Read the model definition and answer for the solid it produces. Units are mm, in the model's axes. A direction names the side the tool comes from. Coordinates: 2 decimals unless noted, no trailing zeros. Order: outer loops, then holes, each group sorted by start corner. A loop starts at its lowest first (then second) coordinate and runs counter-clockwise, first axis right, second up. Notation, with made-up numbers: M -27.5,21.5 L -4.5,21.5 A9 ccw -4.5,27.5 Z; hole C 75,10.25 d10. An arc over 180 degrees is marked long. Use a Markdown table: item, result. Add a question column.
1) The mould has two halves that part along X. Classify faces 3 (the face through (-50.48, 46.61, -21.04)), 4 (the face through (-26.15, 87.218, -26.038)), 5 (the face through (-9.352, 54.274, -25.475)): released by +X, released by -X, zero draft, split by the parting line, or undercut.
2) Find the intervals of material crossed by probe 1 along X at (y, z) = (87.5, -24.5); probe 2 along Y at (x, z) = (-34.5, -22.75); probe 3 along Z at (x, y) = (-10, 94), in increasing order. Write a range as [from, to].
3) Find section B-B on z = -21.5. Write down the section's boundary in (x, y), plus the area to 3 significant figures.
4) Each of these flat-tipped pins is pushed along its axis until it touches: pin 1 Ø5 at (x, y) = (-19, 80.5) entering from -Z; pin 2 Ø5 at (x, y) = (-16.08, 55.44) entering from -Z; pin 3 Ø3 at (x, z) = (-44, -26.5) entering from -Y. Where does it stop, or does it pass through?
5) Find section A-A on z = -27. Write down the section's boundary in (x, y).
6) For faces 1 (the face through (-14.835, 58.443, -23.065)), 2 (the face through (-9.314, 87.768, -25.475)), determine the directions among +Z, -Z, +X, -X, +Y, -Y from which every point of the face is accessible in a straight line to the end or side of a thin tool.
Autodesk Inventor part; units mm, degrees
ref_plane "YZ Plane" through (0, 0, 0) normal (1, 0, 0) x (0, 1, 0)
ref_plane "XZ Plane" through (0, 0, 0) normal (0, 1, 0) x (-1, 0, 0)
ref_plane "XY Plane" through (0, 0, 0) normal (0, 0, 1) x (1, 0, 0)
ref_plane "Arbeitsebene15" through (-38.58009, 58.540516, -23.010083) normal (0, 0, 1) x (1, 0, 0)
sketch "Skizze38" plane through (-38.58009, 58.540516, -23.010083) normal (0, 0, 1) x (1, 0, 0)
  circle A0 centre (27, 33.3) radius 3
  circle A1 centre (-8.3, 27) radius 3
  circle A2 centre (-2, -8.3) radius 3
  circle A3 centre (33.3, -2) radius 3
  circle A4 centre (27, -8.3) radius 3
  circle A5 centre (-8.3, -2) radius 3
  circle A6 centre (-2, 33.3) radius 3
  circle A7 centre (33.3, 27) radius 3
  line L0 (27.5, 29.5) -> (-2.5, 29.5)
  arc A8 (29.5, 27.5) -> (27.5, 29.5) centre (27.5, 27.5) ccw
  line L1 (29.5, 27.5) -> (29.5, -2.5)
  arc A9 (27.5, -4.5) -> (29.5, -2.5) centre (27.5, -2.5) ccw
  line L2 (-2.5, -4.5) -> (27.5, -4.5)
  arc A10 (-4.5, -2.5) -> (-2.5, -4.5) centre (-2.5, -2.5) ccw
  line L3 (-4.5, -2.5) -> (-4.5, 27.5)
  arc A11 (-2.5, 29.5) -> (-4.5, 27.5) centre (-2.5, 27.5) ccw
  circle A12 centre (33.5, 33.5) radius 2.5
  circle A13 centre (-8.5, -8.5) radius 2.5
  circle A14 centre (33.5, -8.5) radius 2.5
  circle A15 centre (-8.5, 33.5) radius 2.5
  line L4 (-11.75, -10.5) -> (-11.75, 8.25)
  arc A16 (-11.75, -10.5) -> (-10.5, -11.75) centre (-10.5, -10.5) ccw
  line L5 (8.25, -11.75) -> (-10.5, -11.75)
  line L6 (8.25, -13.877389) -> (8.25, -11.75)
  arc A17 (7.405556, -14.865216) -> (8.25, -13.877389) centre (7.25, -13.877389) ccw
  arc A18 (7.405556, -14.865216) -> (7.6, -17.35) centre (7.6, -16.1) ccw
  line L7 (17.4, -17.35) -> (7.6, -17.35)
  arc A19 (17.4, -17.35) -> (17.594444, -14.865216) centre (17.4, -16.1) ccw
  arc A20 (16.75, -13.877389) -> (17.594444, -14.865216) centre (17.75, -13.877389) ccw
  line L8 (16.75, -11.75) -> (16.75, -13.877389)
  line L9 (35.5, -11.75) -> (16.75, -11.75)
  arc A21 (35.5, -11.75) -> (36.75, -10.5) centre (35.5, -10.5) ccw
  line L10 (36.75, 6.487451) -> (36.75, -10.5)
  arc A22 (36.75, 6.487451) -> (36.55605, 6.521706) centre (36.65, 6.487451) ccw
  arc A23 (31.3, 7.45) -> (36.55605, 6.521706) centre (34.01, 7.45) ccw
  line L11 (31.3, 17.55) -> (31.3, 7.45)
  arc A24 (36.55605, 18.478294) -> (31.3, 17.55) centre (34.01, 17.55) ccw
  arc A25 (36.55605, 18.478294) -> (36.75, 18.512549) centre (36.65, 18.512549) ccw
  line L12 (36.75, 35.5) -> (36.75, 18.512549)
  arc A26 (36.75, 35.5) -> (35.5, 36.75) centre (35.5, 35.5) ccw
  line L13 (18.512549, 36.75) -> (35.5, 36.75)
  arc A27 (18.512549, 36.75) -> (18.478294, 36.55605) centre (18.512549, 36.65) ccw
  arc A28 (17.55, 31.3) -> (18.478294, 36.55605) centre (17.55, 34.01) ccw
  line L14 (7.45, 31.3) -> (17.55, 31.3)
  arc A29 (6.521706, 36.55605) -> (7.45, 31.3) centre (7.45, 34.01) ccw
  arc A30 (6.521706, 36.55605) -> (6.487451, 36.75) centre (6.487451, 36.65) ccw
  line L15 (-10.5, 36.75) -> (6.487451, 36.75)
  arc A31 (-10.5, 36.75) -> (-11.75, 35.5) centre (-10.5, 35.5) ccw
  line L16 (-11.75, 16.75) -> (-11.75, 35.5)
  line L17 (-13.877389, 16.75) -> (-11.75, 16.75)
  arc A32 (-14.865216, 17.594444) -> (-13.877389, 16.75) centre (-13.877389, 17.75) ccw
  arc A33 (-14.865216, 17.594444) -> (-17.35, 17.4) centre (-16.1, 17.4) ccw
  line L18 (-17.35, 7.6) -> (-17.35, 17.4)
  arc A34 (-17.35, 7.6) -> (-14.865216, 7.405556) centre (-16.1, 7.6) ccw
  arc A35 (-13.877389, 8.25) -> (-14.865216, 7.405556) centre (-13.877389, 7.25) ccw
  line L19 (-11.75, 8.25) -> (-13.877389, 8.25)
  line L20 (-2.5, 30.1) -> (27.5, 30.1)
  arc A36 (30.1, 27.5) -> (27.5, 30.1) centre (27.5, 27.5) ccw
  line L21 (30.1, 27.5) -> (30.1, -2.5)
  arc A37 (27.5, -5.1) -> (30.1, -2.5) centre (27.5, -2.5) ccw
  line L22 (27.5, -5.1) -> (-2.5, -5.1)
  arc A38 (-5.1, -2.5) -> (-2.5, -5.1) centre (-2.5, -2.5) ccw
  line L23 (-5.1, -2.5) -> (-5.1, 27.5)
  arc A39 (-2.5, 30.1) -> (-5.1, 27.5) centre (-2.5, 27.5) ccw
  point P0 (38.58009, -58.540516)
  dimension "d425" = 0.6
sketch "Skizze38 outline for Extrusion20" plane through (-38.58009, 58.540516, -23.010083) normal (0, 0, 1) x (1, 0, 0)
  arc A0 (-5.1, -2.5) -> (-2.5, -5.1) centre (-2.5, -2.5) ccw
  line L0 (-5.1, 27.5) -> (-5.1, -2.5)
  arc A1 (-2.5, 30.1) -> (-5.1, 27.5) centre (-2.5, 27.5) ccw
  line L1 (27.5, 30.1) -> (-2.5, 30.1)
  arc A2 (30.1, 27.5) -> (27.5, 30.1) centre (27.5, 27.5) ccw
  line L2 (30.1, -2.5) -> (30.1, 27.5)
  arc A3 (27.5, -5.1) -> (30.1, -2.5) centre (27.5, -2.5) ccw
  line L3 (-2.5, -5.1) -> (27.5, -5.1)
extrude "Extrusion20" add sketch "Skizze38 outline for Extrusion20" against normal blind 5 draft -3
sketch "Skizze39" plane through (-38.58009, 58.540516, -23.010083) normal (0, 0, 1) x (1, 0, 0)
  line L0 (-2.5, -5.1) -> (27.5, -5.1)
  arc A0 (27.5, -5.1) -> (30.1, -2.5) centre (27.5, -2.5) ccw
  line L1 (30.1, -2.5) -> (30.1, 27.5)
  arc A1 (30.1, 27.5) -> (27.5, 30.1) centre (27.5, 27.5) ccw
  line L2 (27.5, 30.1) -> (-2.5, 30.1)
  arc A2 (-2.5, 30.1) -> (-5.1, 27.5) centre (-2.5, 27.5) ccw
  line L3 (-5.1, 27.5) -> (-5.1, -2.5)
  arc A3 (-5.1, -2.5) -> (-2.5, -5.1) centre (-2.5, -2.5) ccw
  line L4 (17.5, -12.5) -> (35.5, -12.5)
  line L5 (-10.5, 37.5) -> (35.5, 37.5)
  line L6 (37.5, 35.5) -> (37.5, -10.5)
  line L7 (35.5, -12.5) -> (-10.5, -12.5)
  line L8 (-12.5, -10.5) -> (-12.5, 35.5)
  line L9 (-12.5, 37.5) -> (37.5, -12.5) construction
  line L10 (37.5, 37.5) -> (-12.5, -12.5) construction
  arc A4 (37.5, 35.5) -> (35.5, 37.5) centre (35.5, 35.5) ccw
  arc A5 (37.5, 35.5) -> (35.5, 37.5) centre (35.5, 35.5) ccw
  arc A6 (-10.5, 37.5) -> (-12.5, 35.5) centre (-10.5, 35.5) ccw
  arc A7 (-12.5, -10.5) -> (-10.5, -12.5) centre (-10.5, -10.5) ccw
  arc A8 (35.5, -12.5) -> (37.5, -10.5) centre (35.5, -10.5) ccw
  point P0 (38.58009, -58.540516)
  point P1 (12.5, 12.5)
  point P2 (35.5, -12.5)
  dimension "d428" = 50
  dimension "d429" = 50
  dimension "d430" = 2
extrude "Extrusion21" add sketch "Skizze39" along normal blind 4 contours A3 L3 A2 L2 A1 L1 A0 L0 | L7 A7 L8 A6 L5 A4 L6 A8 L4
sketch "Skizze40" plane through (-38.58009, 58.540516, -19.010083) normal (0, 0, 1) x (1, 0, 0)
  arc A0 (-10.5, 37.5) -> (-12.5, 35.5) centre (-10.5, 35.5) ccw
  line L0 (-12.5, 35.5) -> (-12.5, -10.5)
  arc A1 (-12.5, -10.5) -> (-10.5, -12.5) centre (-10.5, -10.5) ccw
  line L1 (-10.5, -12.5) -> (35.5, -12.5)
  arc A2 (35.5, -12.5) -> (37.5, -10.5) centre (35.5, -10.5) ccw
  line L2 (37.5, -10.5) -> (37.5, 35.5)
  arc A3 (37.5, 35.5) -> (35.5, 37.5) centre (35.5, 35.5) ccw
  line L3 (35.5, 37.5) -> (-10.5, 37.5)
  circle A4 centre (12.5, 12.5) radius 5
  line L4 (-2.5, 20) -> (27.5, 20) construction
  line L5 (27.5, 20) -> (27.5, -8) construction
  line L6 (27.5, -8) -> (-2.5, -8) construction
  line L7 (-2.5, -8) -> (-2.5, 20) construction
  circle A5 centre (2.5, -3.1) radius 1.5
  circle A6 centre (22.5, -3.1) radius 1.5
  point P0 (38.58009, -58.540516)
  dimension "d433" = 10
  dimension "d434" = 30
  dimension "d435" = 28
  dimension "d436" = 15
  dimension "d437" = 25
  dimension "d438" = 25
  dimension "d439" = 7.5
  dimension "d440" = 3
  dimension "d441" = 3
  dimension "d442" = 5
  dimension "d443" = 5
  dimension "d466" = 15.6
  dimension "d467" = 15.6
extrude "Extrusion22" cut sketch "Skizze40" against normal through all contours A4 | A5 | A6
sketch "Skizze41" plane through (-38.58009, 58.540516, -28.010083) normal (0, 0, -1) x (-1, 0, 0)
  circle A0 centre (-12.5, 12.5) radius 5
  circle A1 centre (-4.5, 28.5) radius 1.4
  circle A2 centre (-20.5, 28.5) radius 1.4
  circle A3 centre (-2.5, -3.1) radius 1.5
  circle A4 centre (-22.5, -3.1) radius 1.5
  point P0 (-38.58009, -58.540516)
  point P1 (-3.17813, -4.837961)
  point P2 (-1.82187, -4.837961)
  point P3 (-23.17813, -4.837961)
  point P4 (-21.82187, -4.837961)
  dimension "d456" = 2.8
  dimension "d457" = 2.8
  dimension "d458" = 16
  dimension "d459" = 16
  dimension "d460" = 8
  dimension "d461" = 8
hole "Bohrung10" at (-34.08009, 87.040516, -28.010083) at (-18.08009, 87.040516, -28.010083) at (-36.08009, 55.440516, -28.010083) at (-16.08009, 55.440516, -28.010083) direction (0, 0, 1) diameter 2.8 end through all counterbore diameter 6.5 counterbore depth 8
ref_plane "Arbeitsebene16" through (-38.58009, 58.540516, -24.010083) normal (0, 0, -1) x (-1, 0, 0)
sketch "Skizze44" plane through (-38.58009, 58.540516, -24.010083) normal (0, 0, -1) x (-1, 0, 0)
  circle A0 centre (-12.5, 12.5) radius 5
  circle A1 centre (-12.5, 12.5) radius 16
  point P0 (-38.58009, -58.540516)
  dimension "d472" = 32
extrude "Extrusion25" cut sketch "Skizze44" along normal through all draft 5 contours A0 | A1
equation "\"d_i\" = 40"
equation "\"d_o\" = 40"
equation "\"d_part\" = 50"
equation "\"d6\" = 0"
equation "\"d7\" = 0"
equation "\"d8\" = 0"
equation "\"d9\" = 0"
equation "\"d13\" = 0"
equation "\"d14\" = 0"
equation "\"d20\" = 0"
equation "\"d21\" = 0"
equation "\"d22\" = 0"
equation "\"d23\" = 0"
equation "\"d24\" = 0"
equation "\"d25\" = 3"
equation "\"d26\" = 0"
equation "\"d27\" = 0"
equation "\"d28\" = 0"
equation "\"d29\" = 0"
equation "\"d30\" = 0"
equation "\"d31\" = 0"
equation "\"d32\" = 0"
equation "\"d33\" = 0"
equation "\"d34\" = 0"
equation "\"d46\" = 0"
equation "\"d47\" = 0"
equation "\"d48\" = 0"
equation "\"d50\" = 0"
equation "\"d51\" = 0"
equation "\"d52\" = 0"
equation "\"d53\" = 0"
equation "\"d54\" = 0"
equation "\"d55\" = 0"
equation "\"d56\" = 0"
equation "\"d57\" = 0"
equation "\"d58\" = 0"
equation "\"d59\" = 0"
equation "\"magnet_offset\" = 0"
equation "\"screw_offset\" = 0"
equation "\"mal_puzzle_offset\" = 0"
equation "\"fem_puzzle_offset\" = 0"
properties part number "20_Cube_Adapter_Zstage_manual"
Check result:
| question | item | result |
|---|---|---|
| 1 | face 3 | released by -X |
| 1 | face 4 | undercut |
| 1 | face 5 | released by +X |
| 2 | probe 1 | x = [-43.14, -37.3], [-30.86, -21.3], [-14.86, -9.02] |
| 2 | probe 2 | y = [46.04, 52.6], [58.28, 83.82], [90.26, 96.04] |
| 2 | probe 3 | z = [-23.01, -19.01] |
| 3 | outline | M -51.08,48.04 A2 ccw -49.08,46.04 L -3.08,46.04 A2 ccw -1.08,48.04 L -1.08,94.04 A2 ccw -3.08,96.04 L -49.08,96.04 A2 ccw -51.08,94.04 Z; hole C -36.08,55.44 d6.5; hole C -34.08,87.04 d6.5; hole C -26.08,71.04 d10; hole C -18.08,87.04 d6.5; hole C -16.08,55.44 d6.5 |
| 3 | area | 2,290 mm2 |
| 4 | pin 1 | stops at z = -24.01 |
| 4 | pin 2 | stops at z = -20.01 |
| 4 | pin 3 | stops at y = 54.08 |
| 5 | outline | M -43.47,56.04 A2.39 ccw -41.08,53.65 L -38.79,53.65 A3.25 cw -36.61,58.65 A16.26 cw -35.64,84.19 A3.25 cw -37.02,88.43 L -41.08,88.43 A2.39 ccw -43.47,86.04 Z; M -33.37,53.65 L -18.79,53.65 A3.25 cw -19.21,56.3 A16.26 cw -32.95,56.3 A3.25 cw Z; M -31.14,88.43 A3.25 cw -30.86,86.58 A16.26 cw -21.3,86.58 A3.25 cw -21.02,88.43 Z; M -16.52,84.19 A16.26 cw -15.55,58.65 A3.25 cw -13.37,53.65 L -11.08,53.65 A2.39 ccw -8.69,56.04 L -8.69,86.04 A2.39 ccw -11.08,88.43 L -15.14,88.43 A3.25 cw Z |
| 6 | face 1 | -Z |
| 6 | face 2 | -Z, +X, +Y |
